Can you work these out from the model? Positions are in its coordinate system, mm. Give positions to 0.01 mm unless a question says otherwise; leave off trailing zeros. Write each loop counter-clockwise with the first axis right and the second up, starting at its lowest first coordinate (ties: lowest second). Pieces come first, ordered by that corner, then holes. Notation, with made-up numbers: (4, -21.5) -> (15, -21.5) arc R18 cw to (15, -3.5) -> close; hole circle Ø1 at (-12.75, 86.5). An arc over 180 degrees is marked (long way). One line per item, written item: value.
from build123d import *

# Parameters (mm, degrees)
F0_W           = 76.2
F0_H           = 127
F1_DEPTH       = 25.4
F2_R           = 6.35
F4_D           = 11.50874
F4_CSINK_D     = 23.8252
F4_CSINK_ANGLE = 82
F5_R           = 5.08


with BuildPart() as f1:
    # F0 (on Top) → F1 (new body, symmetric)
    with BuildSketch(Plane.XY):
        Rectangle(F0_W, F0_H)
    extrude(amount=F1_DEPTH, both=True)

    # F2
    f2_edges = [f1.edges().sort_by_distance(p)[0] for p in [
        (38.1, -63.5, 0),
        (38.1, 63.5, 0),
        (-38.1, -63.5, 0),
        (-38.1, 63.5, 0),
    ]]
    fillet(f2_edges, radius=F2_R)

    # F4 (through all)
    with Locations(Plane.XY.offset(25.4)):
        with Locations((0, -25.4), (0, 25.4)):
            CounterSinkHole(F4_D / 2, F4_CSINK_D / 2, counter_sink_angle=F4_CSINK_ANGLE)

    # F5
    f5_edges = [f1.edges().sort_by_distance(p)[0] for p in [
        (38.1, 0, 25.4),
        (38.1, 0, -25.4),
    ]]
    fillet(f5_edges, radius=F5_R)


solid = f1.part
1) I need wall thicknesses on L1, parallel to Y at x = 0, z = 9.5; L2, parallel to X at y = -25, z = 0; L3, parallel to X at y = 25.4, z = -16. Which ranges of each line are inside material? Lowest first, please.
Answer list:
L1: y = -63.5 to -31.15, -19.65 to 19.65, 31.15 to 63.5
L2: x = -38.1 to -5.74, 5.74 to 38.1
L3: x = -38.1 to -5.75, 5.75 to 38.1
2) If we section it at B-B (y = 25.4): Write out the boundary of the cut face in (x, z), and give its area (3 significant figures).
Answer list:
outline: (-38.1, -20.32) arc R5.08 ccw to (-33.02, -25.4) -> (-5.75, -25.4) -> (-5.75, 18.32) -> (-11.91, 25.4) -> (-33.02, 25.4) arc R5.08 ccw to (-38.1, 20.32) -> close; (5.75, -25.4) -> (33.02, -25.4) arc R5.08 ccw to (38.1, -20.32) -> (38.1, 20.32) arc R5.08 ccw to (33.02, 25.4) -> (11.91, 25.4) -> (5.75, 18.32) -> close
area: 3,220 mm^2
3) If we section it at A-A (x = 0): Write out the boundary of the cut face in (y, z).
Answer list:
outline: (-63.5, -20.32) arc R5.08 ccw to (-58.42, -25.4) -> (-31.15, -25.4) -> (-31.15, 18.32) -> (-37.31, 25.4) -> (-58.42, 25.4) arc R5.08 ccw to (-63.5, 20.32) -> close; (-19.65, -25.4) -> (19.65, -25.4) -> (19.65, 18.32) -> (13.49, 25.4) -> (-13.49, 25.4) -> (-19.65, 18.32) -> close; (31.15, -25.4) -> (58.42, -25.4) arc R5.08 ccw to (63.5, -20.32) -> (63.5, 20.32) arc R5.08 ccw to (58.42, 25.4) -> (37.31, 25.4) -> (31.15, 18.32) -> close
4) We'd pull the mould along X, two halves only. Please class faces 1 (the face through (38.1, -1, 0)), 2 (the face through (1.247, 19.782, -3.848)), 3 (the face through (0.445, -61.972, 23.951)): released by +X, released by -X, zero draft, split by the parting line, or undercut.
Answer list:
face 1: released by +X
face 2: undercut
face 3: zero draft
5) Will this pin go through, and if not, where does the flat tip stop? pin 1 (15 mm diameter, centred on x = 0, y = -25.4, fed in from +Z).
Answer list:
pin 1: stops at z = 20.32
6) If we section it at C-C (z = -10): Write out the boundary of the cut face in (x, y), and give its area (3 significant figures).
Answer list:
outline: (-38.1, -57.15) arc R6.35 ccw to (-31.75, -63.5) -> (31.75, -63.5) arc R6.35 ccw to (38.1, -57.15) -> (38.1, 57.15) arc R6.35 ccw to (31.75, 63.5) -> (-31.75, 63.5) arc R6.35 ccw to (-38.1, 57.15) -> close; hole circle Ø11.51 at (0, -25.4); hole circle Ø11.51 at (0, 25.4)
area: 9,430 mm^2
